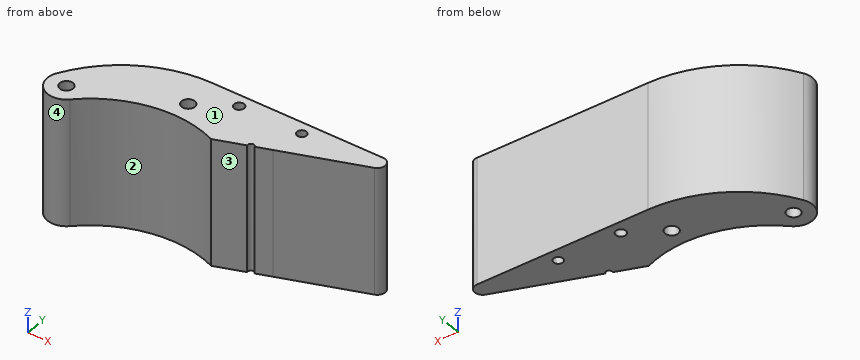
from build123d import *

# Parameters (mm, degrees)
SKETCH_1_R          = 2.1
SKETCH_1_R_2        = 6
EXTRUDE_1_DEPTH     = 40
FILLET_1_R          = 2.5
CUT_EXTRUDE_START   = -40
SKETCH_3_R          = 1.6
SKETCH_3_R_2        = 1.5
SKETCH_3_R_3        = 2.1
CUT_EXTRUDE_2_DEPTH = 40
CUT_EXTRUDE_3_REACH = 89.157
SKETCH_4_R          = 1


with BuildPart() as part:
    # 草图1 → 凸台-拉伸1 (new body)
    # profile 1 of 3: a face of its own
    with BuildSketch(Plane.XY):
        with BuildLine():
            Line((68.135486627, 53), (-0.671642545, 53))
            ThreePointArc((-0.671642545, 53), (15.918389352, 49.295479077), (29.356722765, 38.885684233))
            Line((29.356722765, 38.885684233), (68.135486627, 53))
        make_face()
    # profile 2 of 3: a face of its own
    with BuildSketch(Plane.XY):
        with BuildLine():
            ThreePointArc((29.356722765, 38.885684233), (15.918389352, 49.295479077), (-0.671642545, 53))
            ThreePointArc((-0.671642545, 53), (-20.639649059, 47.500428563), (-34.976092597, 32.552754602))
            ThreePointArc((-34.976092597, 32.552754602), (-28.226351446, 35.515083761), (-23.69848481, 29.69848481))
            ThreePointArc((-23.69848481, 29.69848481), (-24.155207625, 27.402384191), (-25.45584416, 25.455844085))
            ThreePointArc((-25.45584416, 25.455844085), (-6.992802508, 35.314313148), (13.833943007, 33.235854448))
            Line((13.833943007, 33.235854448), (29.356722765, 38.885684233))
        make_face()
        with Locations((0, 42)):
            Circle(SKETCH_1_R, mode=Mode.SUBTRACT)
    # profile 3 of 3: a face of its own
    with BuildSketch(Plane.XY):
        with Locations((-29.69848481, 29.69848481)):
            Circle(SKETCH_1_R_2)
        with Locations((-29.69848481, 29.69848481)):
            Circle(SKETCH_1_R, mode=Mode.SUBTRACT)
    extrude(amount=EXTRUDE_1_DEPTH)

    # 圆角1
    fillet_1_edges = [part.edges().sort_by_distance(p)[0] for p in [
        (68.135486627, 53, 20),
    ]]
    fillet(fillet_1_edges, radius=FILLET_1_R)

    # 草图3 → 切除-拉伸2 (cut)
    with BuildSketch(Plane.XY.offset(40).offset(CUT_EXTRUDE_START)):
        with Locations((11, 49)):
            Circle(SKETCH_3_R)
        with Locations((31, 49)):
            Circle(SKETCH_3_R_2)
        with Locations((0, 42)):
            Circle(SKETCH_3_R_3)
    extrude(amount=CUT_EXTRUDE_2_DEPTH, mode=Mode.SUBTRACT)

    # 草图4 → 切除-拉伸3 (cut, up to next)
    with BuildSketch(Plane.XY.offset(40), mode=Mode.PRIVATE) as cut_extrude_3_sk1:
        with Locations((23.833943007, 36.87555679)):
            Circle(SKETCH_4_R)
    cut_extrude_3_tool1 = extrude(cut_extrude_3_sk1.sketch, amount=-CUT_EXTRUDE_3_REACH, mode=Mode.PRIVATE) & part.part
    add(cut_extrude_3_tool1.solids().sort_by_distance((23.833943, 36.875557, 40))[0], mode=Mode.SUBTRACT)


solid = part.part
CAD build for the part. Positions are in the model's coordinates, mm. Face numbers are marked on the shaded views. Give positions to 0.01 mm unless a question says otherwise; leave off trailing zeros. Order: outer loops, then holes, each group sorted by start corner. A loop starts at its lowest first (then second) coordinate and runs counter-clockwise, first axis right, second up. Notation, with made-up numbers: (36, 54) - (89, 54) arc R23 cw to (89, 80) - close; hole circle Ø8 at (-10.5, -31). An arc over 180 degrees is marked (long way). Answer in a Markdown table with one row per item.
1. Saw through at C-C, the plane z = 5. Give the cut face in (x, y), plus the area to 3 significant figures.
Data:
| item | result |
|---|---|
| outline | (-34.98, 32.55) arc R6 ccw to (-25.46, 25.46) arc R36 cw to (13.83, 33.24) - (22.89, 36.53) arc R1 cw to (24.77, 37.22) - (54.81, 48.15) arc R2.5 ccw to (53.96, 53) - (-0.67, 53) arc R39 ccw to start; hole circle Ø4.2 at (-29.7, 29.7); hole circle Ø4.2 at (0, 42); hole circle Ø3.2 at (11, 49); hole circle Ø3 at (31, 49) |
| area | 1,300 mm² |
2. Saw through at D-D, the plane x = 20.5. Give the cut face in (y, z), plus the area to 3 significant figures.
Data:
| item | result |
|---|---|
| outline | (35.66, 0) - (53, 0) - (53, 40) - (35.66, 40) - close |
| area | 694 mm² |
3. Saw through at B-B, the plane x = 10.5. Give the cut face in (y, z).
Data:
| item | result |
|---|---|
| outline | (34.43, 0) - (47.48, 0) - (47.48, 40) - (34.43, 40) - close; (50.52, 0) - (53, 0) - (53, 40) - (50.52, 40) - close |
4. Pull direction X, two halves, no side cores. Call the marked faces 1, 2, 3 and 4: pulls with the +X half, pulls with the -X half, needs draft (parallel to the pull), parting line crosses it, or undercut.
Data:
| item | result |
|---|---|
| face 1 | needs draft |
| face 2 | undercut |
| face 3 | pulls with the +X half |
| face 4 | parting line crosses it |
5. Saw through at A-A, the plane y = 35. Give the cut face in (x, z) (3 decimals), plus the area to 3 significant figures.
Data:
| item | result |
|---|---|
| outline | (-33.535, 0) - (-8.426, 0) - (-8.426, 40) - (-33.535, 40) - close; (8.426, 0) - (18.681, 0) - (18.681, 40) - (8.426, 40) - close |
| area | 1,410 mm² |
6. Probe probe 1 along Y at (x, z) = (0, 17); probe 2 along Y at (x, z) = (11, 16); probe 3 along X at (y, z) = (28, 2.5). List the from-to ranges inside material, lowest first. Write a range as [from, to].
Data:
| item | result |
|---|---|
| probe 1 | y = [36, 39.9], [44.1, 53] |
| probe 2 | y = [34.28, 47.4], [50.6, 53] |
| probe 3 | x = [-35.45, -30.93], [-28.46, -22.63] |
7. Flat gauge pins, fed straight in: pin 1 (3 mm diameter, centred on x = 30, y = 42, fed in from -Z); pin 2 (2 mm diameter, centred on y = 29, z = 20, fed in from +X); pin 3 (12 mm diameter, centred on x = 36, z = 6.5, fed in from -Y); pin 4 (4 mm diameter, centred on x = -29.7, y = 29.7, fed in from -Z). Where does each tip first touch, or does it go through?
Data:
| item | result |
|---|---|
| pin 1 | stops at z = 0 |
| pin 2 | stops at x = -19.9 |
| pin 3 | stops at y = 39.12 |
| pin 4 | passes through |
